Part model, mm, in its own coordinate system. Face numbers are marked on the shaded views. Coordinates: 2 decimals unless noted, no trailing zeros. Loops run counter-clockwise (first coordinate to the right, second up) from the corner with the lowest first, then second, coordinate; pieces in that order, holes last. Notation, with made-up numbers: M 20,33.5 L 27,33.5 A15 ccw 27,47.5 Z; hole C 46,31.5 d10. An arc over 180 degrees is marked long. Answer as a JSON object with one key per item and string values. Group by question number.
1. Saw through at B-B on x = 3.25. Write the cut outline in (y, z), then the cut area to 3 significant figures.
2. Saw through at A-A on x = 14. Write the cut outline in (y, z), then the cut area to 3 significant figures.
3. Drop flat-ended pins along their axis: pin 1 Ø2 at (y, z) = (12.5, 4) entering from -X; pin 2 Ø1.5 at (y, z) = (12.5, 4) entering from -X. Give the stop position or say it passes through.
4. Mould opens along X. For the marked faces 1, 2, 3 and 4 say: released by +X, released by -X, zero draft, split by the parting line, or undercut.
5. Drill centre lines: L1, parallel to Y at x = 23, z = 4; L2, parallel to Z at x = 4, y = 12.5; L3, parallel to Y at x = 5.75, z = 3.25. Where is each one in solid material? Low to high.
from build123d import *

# Parameters (mm, degrees)
SKETCH_1_W          = 28
SKETCH_1_H          = 60
EXTRUDE_1_DEPTH     = 8
SKETCH_2_R          = 2.5
CUT_EXTRUDE_1_DEPTH = 67.693328002
M3X0_5_1_D          = 2.5
M3X0_5_1_DEPTH      = 7.5
M3X0_5_1_TIP        = 0.751075774
M3X0_5_2_D          = 2.5
M3X0_5_2_DEPTH      = 7.5
M3X0_5_2_TIP        = 0.751075774


with BuildPart() as part:
    # ｽｹｯﾁ1 → ﾎﾞｽ - 押し出し1 (new body)
    with BuildSketch(Plane.XY):
        with Locations((14, 30)):
            Rectangle(SKETCH_1_W, SKETCH_1_H)
    extrude(amount=EXTRUDE_1_DEPTH)

    # ｽｹｯﾁ2 → ｶｯﾄ - 押し出し1 (cut, through all)
    with BuildSketch(Plane.XY.offset(8)):
        with Locations((14, 10)):
            Circle(SKETCH_2_R)
    extrude(amount=-CUT_EXTRUDE_1_DEPTH, mode=Mode.SUBTRACT)

    # M3x0.5 ねじ穴1
    with Locations(Plane(origin=(0, 47.5, 4), x_dir=(0, 0, -1), z_dir=(-1, 0, 0))):
        with Locations((0, 0), (0, 35)):
            Hole(M3X0_5_1_D / 2, depth=M3X0_5_1_DEPTH)
            with Locations((0, 0, -(M3X0_5_1_DEPTH + M3X0_5_1_TIP / 2))):  # 118° drill point
                Cone(0, M3X0_5_1_D / 2, M3X0_5_1_TIP, mode=Mode.SUBTRACT)

    # M3x0.5 ねじ穴2
    with Locations(Plane(origin=(28, 47.5, 4), x_dir=(0, 0, 1), z_dir=(1, 0, 0))):
        with Locations((0, 0), (0, 35)):
            Hole(M3X0_5_2_D / 2, depth=M3X0_5_2_DEPTH)
            with Locations((0, 0, -(M3X0_5_2_DEPTH + M3X0_5_2_TIP / 2))):  # 118° drill point
                Cone(0, M3X0_5_2_D / 2, M3X0_5_2_TIP, mode=Mode.SUBTRACT)


solid = part.part
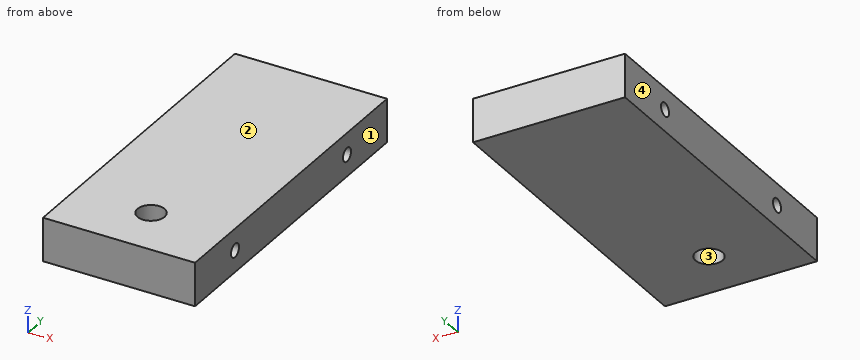
Outcome:
{
 "1": {"outline": "M 0,0 L 60,0 L 60,8 L 0,8 Z; hole C 12.5,4 d2.5; hole C 47.5,4 d2.5", "area": "470 mm²"},
 "2": {"outline": "M 0,0 L 7.5,0 L 7.5,8 L 0,8 Z; M 12.5,0 L 60,0 L 60,8 L 12.5,8 Z", "area": "440 mm²"},
 "3": {"pin 1": "stops at x = 7.65", "pin 2": "stops at x = 7.8"},
 "4": {"face 1": "released by +X", "face 2": "zero draft", "face 3": "undercut", "face 4": "released by -X"},
 "5": {"L1": "y = 0 to 11.25, 13.75 to 46.25, 48.75 to 60", "L2": "z = 0 to 2.75, 5.25 to 8", "L3": "y = 0 to 11.5, 13.5 to 46.5, 48.5 to 60"}
}
